The model under review builds one solid part; all positions refer to its coordinate system, in mm. Face numbers are marked on the shaded views. A direction names the side the tool comes from. Round coordinates to 2 decimals unless told otherwise and drop trailing zeros. Loops run counter-clockwise (first coordinate to the right, second up) from the corner with the lowest first, then second, coordinate; pieces in that order, holes last. Notation, with made-up numbers: (13, 13) -> (34, 13) arc R13 ccw to (34, 33) -> close; hole circle Ø2 at (47.25, 18.25). An arc over 180 degrees is marked (long way). Use a Markdown table: item, result. Add a question column.
1) Wall thickness on probe 1 along Y at (x, z) = (-11.5, -20.5); probe 2 along X at (y, z) = (1.5, -21); probe 3 along X at (y, z) = (0.6, -15.5): over which ranges is each line inside the solid? List them lowest first.
2) Mouldability with a two-part tool opening along Y and no side actions: class the marked faces 1, 2, 3 and 4 as released by +Y, released by -Y, zero draft, split by the parting line, or undercut.
3) Consider section B-B on y = 10. Give the boundary of the cut face in (x, z).
4) Consider section C-C on x = -8.5. Give the boundary of the cut face in (y, z), plus the area to 3 significant figures.
5) Insertion check: pin 1 (1 mm diameter, centred on y = 2.5, z = -7.5, fed in from +X); pin 2 (4 mm diameter, centred on y = 9.5, z = -21.5, fed in from -X); pin 3 (0.5 mm diameter, centred on x = -27, z = -29.5, fed in from +Y). Each pin has a flat end and moves straight along its axis. Give the tip position at first contact, or say it passes through.
6) Consider section A-A on x = 2.5. Give the boundary of the cut face in (y, z).
7) For the marked faces 5, 6 and 7, list the 3-axis set-ups (+Z, -Z, +X, -X, +Y, -Y) from which the entire face can be reached by the end or side of a thin tool; tool diameter is ignored.
8) Consider section D-D on z = -15.5. Give the boundary of the cut face in (x, y), plus the area to 3 significant figures.
Autodesk Inventor part; units mm, degrees
ref_plane "YZ Plane" through (0, 0, 0) normal (1, 0, 0) x (0, 1, 0)
ref_plane "XZ Plane" through (0, 0, 0) normal (0, 1, 0) x (-1, 0, 0)
ref_plane "XY Plane" through (0, 0, 0) normal (0, 0, 1) x (1, 0, 0)
sketch "Esboço1" plane through (0, 0, 0) normal (0, 1, 0) x (-1, 0, 0)
  line L0 (0, 0) -> (25, 0)
  line L1 (25, 0) -> (25, -30)
  line L2 (25, -30) -> (0, -30)
  line L3 (0, -30) -> (0, 0)
  dimension "d0" = 25
  dimension "d1" = 30
extrude "Extrusão1" add sketch "Esboço1" along normal blind 15
shell "Casca1" thickness 1 removed faces 1 at (-8.3333, 15, -10)
sketch "Esboço4" plane through (-24, 1, -1) normal (0, 1, 0) x (1, 0, 0)
  line L0 (24, 29) -> (-1, 29)
  line L1 (-1, 29) -> (-1, -1)
  circle A0 centre (11.5, 14.5) radius 3.5
  point P0 (24, -1)
  point P1 (1, 29)
  dimension "d17" = 7
  dimension "d20" = 12.5
  dimension "d21" = 14.5
extrude "Extrusão4" cut sketch "Esboço4" against normal blind 5
sketch "Esboço10" plane through (0, 0, 0) normal (0, -1, 0) x (1, 0, 0)
  circle A0 centre (-12.5, -15.5) radius 3.5
  circle A1 centre (-16.5, -23) radius 1.65
  circle A2 centre (-8.5, -23) radius 1.65
  point P0 (0, 0)
  dimension "d72" = 3.3
  dimension "d73" = 3.3
  dimension "d113" = 7.5
  dimension "d114" = 4
extrude "Extrusão10" cut sketch "Esboço10" against normal blind 10 contours A1 | A2
sketch "Esboço11" plane through (0, 0, -30) normal (0, 0, -1) x (-1, 0, 0)
  line L0 (1, 1) -> (1, 15)
  line L1 (24, 1) -> (24, 15)
  line L2 (1, 1) -> (24, 1)
  line L3 (24, 1) -> (24, 14)
  line L4 (24, 14) -> (1, 14)
  line L5 (1, 14) -> (1, 1)
  line L6 (0, 15) -> (25, 15)
  point P0 (0, 0)
  dimension "d80" = 1
extrude "Extrusão11" cut sketch "Esboço11" against normal blind 10 contours L0 L4 L1 L2
sketch "Esboço12" plane through (-1, 1, -1) normal (0, 0, -1) x (-1, 0, 0)
  line L0 (0, 13) -> (0, 14)
  line L1 (0, 14) -> (23, 14)
  line L2 (23, 14) -> (23, 13)
  line L3 (23, 13) -> (0, 13)
  line L4 (0, 13) -> (0, 14)
  point P0 (-1, -1)
extrude "Extrusão12" add sketch "Esboço12" along normal up to surface (28 mm away)
sketch "Esboço13" plane through (0, 0, 0) normal (0, -1, 0) x (1, 0, 0)
  circle A0 centre (-16.5, -23) radius 1.65
  circle A1 centre (-16.5, -23) radius 1.65
  circle A2 centre (-8.5, -23) radius 1.65
  circle A3 centre (-8.5, -23) radius 1.65
  point P0 (0, 0)
extrude "Extrusão13" cut sketch "Esboço13" against normal up to surface (15 mm away)
sketch "Esboço14" plane through (0, 0, -30) normal (0, 0, -1) x (-1, 0, 0)
  line L0 (0, 0.7381) -> (-5, 0.7381)
  line L1 (-5, 0.7381) -> (-5, 14)
  line L2 (-5, 14) -> (0, 14)
  line L3 (0, 14) -> (0, 0.7381)
  line L4 (1, 14) -> (24, 14)
  line L5 (25, 0) -> (25, 15)
  line L6 (25, 1) -> (30, 1)
  line L7 (30, 1) -> (30, 14)
  line L8 (30, 14) -> (25, 14)
  line L9 (25, 14) -> (25, 1)
  line L10 (24, 1) -> (1, 1)
  point P0 (0, 0)
  dimension "d88" = 5
  dimension "d89" = 0
  dimension "d90" = 5
  dimension "d91" = 0
  dimension "d92" = 0
extrude "Extrusão14" add sketch "Esboço14" against normal blind 1
sketch "Esboço15" plane through (0, 0, -30) normal (0, 0, -1) x (-1, 0, 0)
  circle A0 centre (27.5, 7.5) radius 1.5
  circle A1 centre (-2.5, 7.2381) radius 1.5
  line L0 (25, 1) -> (30, 1)
  line L1 (0, 0.7381) -> (-5, 0.7381)
  line L2 (-5, 0.7381) -> (-5, 14)
  line L3 (30, 1) -> (30, 14)
  point P0 (0, 0)
  dimension "d95" = 3
  dimension "d96" = 3
  dimension "d97" = 6.5
  dimension "d98" = 6.5
  dimension "d99" = 2.5
  dimension "d100" = 2.5
extrude "Extrusão15" cut sketch "Esboço15" against normal blind 1
fillet "Arredondamento4" radius 1.5 1 edges at (-12.5, 15, 0)
sketch "Esboço16" plane through (-25, 0, 0) normal (0, 0, 1) x (1, 0, 0)
  line L0 (5, 10.5) -> (20, 10.5)
  line L1 (20, 10.5) -> (20, 8.5)
  line L2 (20, 8.5) -> (5, 8.5)
  line L3 (5, 8.5) -> (5, 10.5)
  line L4 (25, 0) -> (25, 13.5)
  line L5 (0, 13.5) -> (25, 13.5)
  dimension "d115" = 15
  dimension "d116" = 2
  dimension "d117" = 5
  dimension "d118" = 3
extrude "Extrusão16" cut sketch "Esboço16" against normal blind 1
properties part number "Caixa do sensor de temperatura"
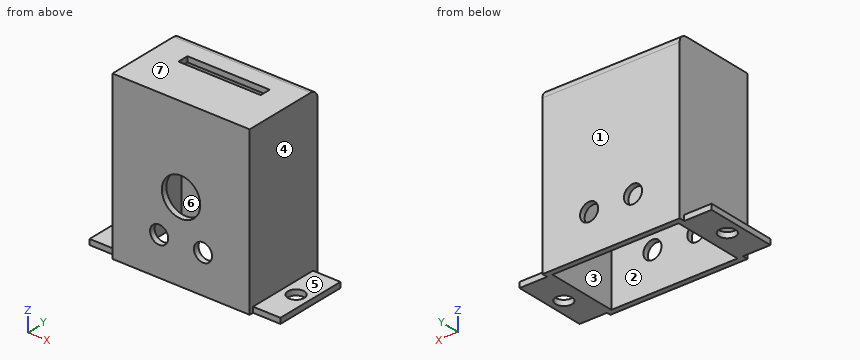
Result set:
| question | item | result |
|---|---|---|
| 1 | probe 1 | 0 to 1, 14 to 15 |
| 1 | probe 2 | -25 to -24, -1 to 0 |
| 1 | probe 3 | -25 to -16, -9 to 0 |
| 2 | face 1 | released by +Y |
| 2 | face 2 | undercut |
| 2 | face 3 | undercut |
| 2 | face 4 | zero draft |
| 3 | outline | (-30, -30) -> (-24, -30) -> (-24, -1) -> (-20, -1) -> (-20, 0) -> (-25, 0) -> (-25, -29) -> (-30, -29) -> close; (-5, -1) -> (-1, -1) -> (-1, -30) -> (5, -30) -> (5, -29) -> (0, -29) -> (0, 0) -> (-5, 0) -> close |
| 4 | outline | (0, -30) -> (1, -30) -> (1, -24.65) -> (0, -24.65) -> close; (0, -21.35) -> (1, -21.35) -> (1, -1) -> (8.5, -1) -> (8.5, 0) -> (0, 0) -> close; (10.5, -1) -> (14, -1) -> (14, -21.35) -> (15, -21.35) -> (15, -1.5) arc R1.5 ccw to (13.5, 0) -> (10.5, 0) -> close; (14, -30) -> (15, -30) -> (15, -24.65) -> (14, -24.65) -> close |
| 4 | area | 63.9 mm2 |
| 5 | pin 1 | x = 0 |
| 5 | pin 2 | x = -25 |
| 5 | pin 3 | y = 14 |
| 6 | outline | (0.74, -30) -> (5.74, -30) -> (5.74, -29) -> (0.74, -29) -> close; (8.74, -30) -> (14, -30) -> (14, -29) -> (8.74, -29) -> close |
| 7 | face 5 | +Z, +X, +Y, -Y |
| 7 | face 6 | -Z |
| 7 | face 7 | +Z, +X, -X, +Y, -Y |
| 8 | outline | (-25, 0) -> (-16, 0) -> (-16, 1) -> (-24, 1) -> (-24, 14) -> (-1, 14) -> (-1, 1) -> (-9, 1) -> (-9, 0) -> (0, 0) -> (0, 15) -> (-25, 15) -> close |
| 8 | area | 69.0 mm2 |
